Geometry: final body of the model. Coordinates: model frame, mm. A direction names the side the tool comes from. Round coordinates to 2 decimals unless told otherwise and drop trailing zeros. Loops run counter-clockwise (first coordinate to the right, second up) from the corner with the lowest first, then second, coordinate; pieces in that order, holes last. Notation, with made-up numbers: (-23.75, -9.5) -> (25.25, -9.5) arc R18 cw to (25.25, 8.5) -> close; hole circle Ø3 at (71.25, 73). An arc over 180 degrees is marked (long way). Answer in a Markdown table with one row per item.
```python
from build123d import *

# Parameters (mm, degrees)
F1_DEPTH = 12.7
F3_D     = 3.81


# Not quite as in the source:
# - a feature names something its author has since deleted; it is built from what else it names


with BuildPart() as f1:
    # F0 (on Front) → F1 (new body)
    with BuildSketch(Plane.XZ):
        with BuildLine():
            Line((-0.6058157035, 13.9202102855), (-0.6058157035, 41.9618102855))
            Line((-0.6058157035, 41.9618102855), (-2.6976561639, 41.9618102855))
            Line((-2.6976561639, 41.9618102855), (-72.5894157035, 41.9618102855))
            Line((-72.5894157035, 41.9618102855), (-72.5894157035, 29.5285102855))
            Line((-72.5894157035, 29.5285102855), (-59.4971985196, 29.5285102855))
            Line((-59.4971985196, 29.5285102855), (-56.8120155754, 29.5285102855))
            ThreePointArc((-56.8120155754, 29.5285102855), (-32.5437541307, 40.9543939264), (-15.88096278, 19.934148568))
            ThreePointArc((-15.88096278, 19.934148568), (-16.0956571498, 16.8969773161), (-16.7354703496, 13.9202102855))
            Line((-16.7354703496, 13.9202102855), (-0.6058157035, 13.9202102855))
        make_face()
        with BuildLine():
            Line((-72.5894157035, 13.9202102855), (-58.2064552105, 13.9202102855))
            ThreePointArc((-58.2064552105, 13.9202102855), (-59.0599250667, 20.1458261131), (-58.0845479883, 26.3535102855))
            Line((-58.0845479883, 26.3535102855), (-59.4971985196, 26.3535102855))
            Line((-59.4971985196, 26.3535102855), (-72.5894157035, 26.3535102855))
            Line((-72.5894157035, 26.3535102855), (-72.5894157035, 13.9202102855))
        make_face()
        with BuildLine():
            Line((-20.7389292415, 13.9202102855), (-16.7354703496, 13.9202102855))
            ThreePointArc((-16.7354703496, 13.9202102855), (-16.0956571498, 16.8969773161), (-15.88096278, 19.934148568))
            ThreePointArc((-15.88096278, 19.934148568), (-32.5437541307, 40.9543939264), (-56.8120155754, 29.5285102855))
            Line((-56.8120155754, 29.5285102855), (-52.8308911926, 29.5285102855))
            Line((-52.8308911926, 29.5285102855), (-52.8308911926, 28.8896496238))
            ThreePointArc((-52.8308911926, 28.8896496238), (-32.8325970751, 37.098470972), (-19.69096278, 19.934148568))
            ThreePointArc((-19.69096278, 19.934148568), (-19.9549136205, 16.881867152), (-20.7389292415, 13.9202102855))
        make_face()
        with BuildLine():
            ThreePointArc((-58.2064552105, 13.9202102855), (-37.47096278, -1.655851432), (-16.7354703496, 13.9202102855))
            Line((-16.7354703496, 13.9202102855), (-20.7389292415, 13.9202102855))
            ThreePointArc((-20.7389292415, 13.9202102855), (-37.47096278, 2.154148568), (-54.2029963185, 13.9202102855))
            Line((-54.2029963185, 13.9202102855), (-58.2064552105, 13.9202102855))
        make_face()
        with BuildLine():
            ThreePointArc((-58.0845479883, 26.3535102855), (-59.0599250667, 20.1458261131), (-58.2064552105, 13.9202102855))
            Line((-58.2064552105, 13.9202102855), (-54.2029963185, 13.9202102855))
            ThreePointArc((-54.2029963185, 13.9202102855), (-55.249646191, 20.1505190165), (-54.0516803501, 26.3535102855))
            Line((-54.0516803501, 26.3535102855), (-58.0845479883, 26.3535102855))
        make_face()
    extrude(amount=F1_DEPTH)

    # F3 (through all)
    with Locations(Plane(origin=(0, 0, 0), x_dir=(1, 0, 0), z_dir=(0, 0, -1))):
        with Locations((-68.9064157035, 6.35), (-4.2888157035, 6.35)):
            Hole(F3_D / 2)


solid = f1.part
```
Item 1: Pin query (flat end, axial travel): pin 1 Ø1.5 at (y, z) = (-3.5, 12) entering from +X; pin 2 Ø2.5 at (x, y) = (-68.91, -6.35) entering from +Z; pin 3 Ø4 at (x, y) = (-66, -8.5) entering from -Z; pin 4 Ø6 at (x, y) = (-60.5, -4.5) entering from -Z. Return the tip coordinate at first contact, or that it passes through.
Answer:
| item | result |
|---|---|
| pin 1 | stops at x = -17.11 |
| pin 2 | passes through |
| pin 3 | stops at z = 13.92 |
| pin 4 | stops at z = 11.87 |
Item 2: Draft query along Z for faces 1 (the face through (-63, -6, 29.529)), 2 (the face through (-63, -6, 26.354)), 3 (the face through (-37.86, -6.261, -1.652)), 4 (the face through (-70.666, -5.62, 20.224)). Return one class per face: pulls with the +Z half, pulls with the -Z half, needs draft (parallel to the pull), parting line crosses it, or undercut.
Answer:
| item | result |
|---|---|
| face 1 | undercut |
| face 2 | undercut |
| face 3 | pulls with the -Z half |
| face 4 | needs draft |
Item 3: Cut plane A-A (x = -66). Output: boundary loops of the cut face in (y, z), then the cut area to 3 significant figures.
Answer:
| item | result |
|---|---|
| outline | (-12.7, 13.92) -> (0, 13.92) -> (0, 26.35) -> (-12.7, 26.35) -> close; (-12.7, 29.53) -> (0, 29.53) -> (0, 41.96) -> (-12.7, 41.96) -> close |
| area | 316 mm² |
Item 4: Reachability of faces 5 (the face through (-9, -6, 13.92)), 6 (the face through (-65, -6, 13.92)), 7 (the face through (-72.589, -6, 20)) from +Z, -Z, +X, -X, +Y, -Y: full face, straight path, thin tool, end or side. Return the list, or none.
Answer:
| item | result |
|---|---|
| face 5 | -Z, +X, +Y, -Y |
| face 6 | -Z, -X, +Y, -Y |
| face 7 | +Z, -Z, -X, +Y, -Y |
Item 5: Cut plane D-D (x = -47.5). Output: boundary loops of the cut face in (y, z), then the cut area to 3 significant figures.
Answer:
| item | result |
|---|---|
| outline | (-12.7, 0.81) -> (0, 0.81) -> (0, 5.25) -> (-12.7, 5.25) -> close; (-12.7, 34.62) -> (0, 34.62) -> (0, 41.96) -> (-12.7, 41.96) -> close |
| area | 150 mm² |
Item 6: Cut plane C-C (y = -1.5). Output: boundary loops of the cut face in (x, z).
Answer:
| item | result |
|---|---|
| outline | (-72.59, 13.92) -> (-58.21, 13.92) arc R21.59 ccw to (-16.74, 13.92) -> (-0.61, 13.92) -> (-0.61, 41.96) -> (-72.59, 41.96) -> (-72.59, 29.53) -> (-52.83, 29.53) -> (-52.83, 28.89) arc R17.78 cw (long way) to (-54.05, 26.35) -> (-72.59, 26.35) -> close |
Item 7: Cut plane B-B (y = -6.35). Output: boundary loops of the cut face in (x, z), then the cut area to 3 significant figures.
Answer:
| item | result |
|---|---|
| outline | (-72.59, 13.92) -> (-70.81, 13.92) -> (-70.81, 26.35) -> (-72.59, 26.35) -> close; (-72.59, 29.53) -> (-70.81, 29.53) -> (-70.81, 41.96) -> (-72.59, 41.96) -> close; (-67, 13.92) -> (-58.21, 13.92) arc R21.59 ccw to (-16.74, 13.92) -> (-6.19, 13.92) -> (-6.19, 41.96) -> (-67, 41.96) -> (-67, 29.53) -> (-52.83, 29.53) -> (-52.83, 28.89) arc R17.78 cw (long way) to (-54.05, 26.35) -> (-67, 26.35) -> close; (-2.38, 13.92) -> (-0.61, 13.92) -> (-0.61, 41.96) -> (-2.38, 41.96) -> close |
| area | 1,240 mm² |
Item 8: Line query: probe 1 along Z at (x, y) = (-62, -10.5); probe 2 along Z at (x, y) = (-8, -5.5); probe 3 along Y at (x, z) = (-4, 40.5). Output: solid intervals per line, ascending. Write a range as [from, to].
Answer:
| item | result |
|---|---|
| probe 1 | z = [13.92, 26.35], [29.53, 41.96] |
| probe 2 | z = [13.92, 41.96] |
| probe 3 | y = [-12.7, -8.23], [-4.47, 0] |
